Build history of the part. All positions in model axes, mm. A direction names the side the tool comes from. Round coordinates to 2 decimals unless told otherwise and drop trailing zeros. Write each loop counter-clockwise with the first axis right and the second up, starting at its lowest first coordinate (ties: lowest second). Pieces come first, ordered by that corner, then holes. Notation, with made-up numbers: (71.25, -1) -> (104.25, -1) arc R24 ccw to (104.25, 30) -> close; hole circle Ø8 at (32, -36). An arc over 180 degrees is marked (long way). Answer in a Markdown table with one row per item.
```python
from build123d import *

# Parameters (mm, degrees)
BOSS_EXTRUDE1_DEPTH = 20
SKETCH4_R           = 6
CUT_EXTRUDE11_DEPTH = 142.431949953
CUT_EXTRUDE12_START = 10
SKETCH4_13_R        = 10
SKETCH4_13_R_2      = 6
CUT_EXTRUDE12_DEPTH = 132.431949953


with BuildPart() as part:
    # Sketch1 → Boss-Extrude1 (new, symmetric)
    with BuildSketch(Plane.XY):
        with BuildLine():
            Line((0, 0), (0, 40))
            Line((0, 40), (74.844322004, 40.582598355))
            ThreePointArc((74.844322004, 40.582598355), (78.147309148, 40.334012976), (81.36396939, 39.543686675))
            Line((81.36396939, 39.543686675), (131.272793878, 22.792096484))
            ThreePointArc((131.272793878, 22.792096484), (133.247397074, 21.335468314), (134, 19))
            Line((134, 19), (134, 0))
            Line((134, 0), (0, 0))
        make_face()
    extrude(amount=BOSS_EXTRUDE1_DEPTH, both=True)

    # Sketch4 → Cut-Extrude11 (cut, through all)
    with BuildSketch(Plane(origin=(0, 0, 0), x_dir=(1, 0, 0), z_dir=(0, 1, 0))):
        with Locations(Location((20, 0, 0), (0, 0, 180))):
            Circle(SKETCH4_R)
        with Locations((105, 0)):
            Circle(SKETCH4_R)
    extrude(amount=CUT_EXTRUDE11_DEPTH, mode=Mode.SUBTRACT)

    # Sketch4_13 → Cut-Extrude12 (cut, through all)
    # profile 1 of 2: a face of its own
    with BuildSketch(Plane(origin=(0, 0, 0), x_dir=(1, 0, 0), z_dir=(0, 1, 0)).offset(CUT_EXTRUDE12_START)):
        with Locations(Location((20, 0, 0), (0, 0, 180))):
            Circle(SKETCH4_13_R)
        with Locations(Location((20, 0, 0), (0, 0, 270))):
            Circle(SKETCH4_13_R_2, mode=Mode.SUBTRACT)
    # profile 2 of 2: a face of its own
    with BuildSketch(Plane(origin=(0, 0, 0), x_dir=(1, 0, 0), z_dir=(0, 1, 0)).offset(CUT_EXTRUDE12_START)):
        with Locations((105, 0)):
            Circle(SKETCH4_13_R)
        with Locations(Location((105, 0, 0), (0, 0, 270))):
            Circle(SKETCH4_13_R_2, mode=Mode.SUBTRACT)
    extrude(amount=CUT_EXTRUDE12_DEPTH, mode=Mode.SUBTRACT)


solid = part.part
```
Q1. Two-plate mould, pull along Z, no slides. Class faces 1 (the cylindrical face through (10.46, 24.91, 3)), 2 (the flat face through (0, 20, 0)), 3 (the flat face through (68, 21, -20)): released by +Z, released by -Z, zero draft, split by the parting line, or undercut.
A:
| item | result |
|---|---|
| face 1 | undercut |
| face 2 | zero draft |
| face 3 | released by -Z |
Q2. Drop flat-ended pins along their axis: P1, Ø6, axis at y = 25, z = -3, coming from the +X side; P2, Ø9.5, axis at x = 105, z = 0, coming from the +Y side; P3, Ø22, axis at x = 104, z = 4.5, coming from the +Y side. Give the stop position or say it passes through.
A:
| item | result |
|---|---|
| P1 | x = 132.65 |
| P2 | through |
| P3 | y = 35.64 |
Q3. Saw through at D-D on z = 13. Write the cut outline in (x, y).
A:
| item | result |
|---|---|
| outline | (0, 0) -> (134, 0) -> (134, 19) arc R4 ccw to (131.27, 22.79) -> (81.36, 39.54) arc R20 ccw to (74.84, 40.58) -> (0, 40) -> close |
Q4. Saw through at B-B on z = 2.5. Write the cut outline in (x, y).
A:
| item | result |
|---|---|
| outline | (0, 0) -> (14.55, 0) -> (14.55, 10) -> (10.32, 10) -> (10.32, 40.08) -> (0, 40) -> close; (25.45, 0) -> (99.55, 0) -> (99.55, 10) -> (95.32, 10) -> (95.32, 34.86) -> (81.36, 39.54) arc R20 ccw to (74.84, 40.58) -> (29.68, 40.23) -> (29.68, 10) -> (25.45, 10) -> close; (110.45, 0) -> (134, 0) -> (134, 19) arc R4 ccw to (131.27, 22.79) -> (114.68, 28.36) -> (114.68, 10) -> (110.45, 10) -> close |
Q5. Saw through at A-A on x = 105. Write the cut outline in (y, z).
A:
| item | result |
|---|---|
| outline | (0, -20) -> (31.61, -20) -> (31.61, -10) -> (10, -10) -> (10, -6) -> (0, -6) -> close; (0, 6) -> (10, 6) -> (10, 10) -> (31.61, 10) -> (31.61, 20) -> (0, 20) -> close |
Q6. Which spindle directions (+Z, -Z, +X, -X, +Y, -Y) get a long thin tool onto all of the face, cutting with end or side? Do faces 4 (the cylindrical face through (95, 20, 0)), 5 (the flat face through (134, 10, 0)). Say none if no direction does.
A:
| item | result |
|---|---|
| face 4 | +Y |
| face 5 | +Z, -Z, +X, +Y, -Y |
Q7. Saw through at C-C on y = 4.5. Write the cut outline in (x, z).
A:
| item | result |
|---|---|
| outline | (0, -20) -> (134, -20) -> (134, 20) -> (0, 20) -> close; hole circle Ø12 at (20, 0); hole circle Ø12 at (105, 0) |
Q8. Wall check: line 1 (X direction, y = 18.75, z = 0); line 2 (X direction, y = 7.5, z = 0); line 3 (Z direction, x = 105, y = 7.5). Give the ranges that are in metal, low to high. Write a range as [from, to].
A:
| item | result |
|---|---|
| line 1 | [0, 10], [30, 95], [115, 134] |
| line 2 | [0, 14], [26, 99], [111, 134] |
| line 3 | [-20, -6], [6, 20] |
